Model file for the job. Use its own axes, mm. Face numbers are marked on the shaded views. A direction names the side the tool comes from. Round coordinates to 2 decimals unless told otherwise and drop trailing zeros. Order: outer loops, then holes, each group sorted by start corner. A loop starts at its lowest first (then second) coordinate and runs counter-clockwise, first axis right, second up. Notation, with made-up numbers: (-40, 44.25) - (7, 44.25) arc R12 cw to (7, 55.25) - close; hole circle Ø6 at (5, 13.25). An arc over 180 degrees is marked (long way). Write item = value, one per line. Start each with the question number.
from build123d import *

# Parameters (mm, degrees)
SKETCH_2_W          = 75
SKETCH_2_H          = 40
EXTRUDE_1_DEPTH     = 2
SKETCH_3_R          = 5.05
SKETCH_3_R_2        = 1.25
CUT_EXTRUDE_1_DEPTH = 86.023526156
FILLET_1_R          = 20
SKETCH_7_W          = 2
SKETCH_7_H          = 40
EXTRUDE_3_DEPTH     = 12
SKETCH_8_R          = 1.5
CUT_EXTRUDE_2_DEPTH = 10


with BuildPart() as part:
    # 草图2 → 凸台-拉伸1 (new body)
    with BuildSketch(Plane.XY):
        with Locations((37.5, 20)):
            Rectangle(SKETCH_2_W, SKETCH_2_H)
    extrude(amount=EXTRUDE_1_DEPTH)

    # 草图3 → 切除-拉伸1 (cut, through all)
    with BuildSketch(Plane(origin=(0, 0, 0), x_dir=(-1, 0, 0), z_dir=(0, 0, -1))):
        with Locations((-26, 20)):
            Circle(SKETCH_3_R)
        with Locations((-16, 10.202041029)):
            Circle(SKETCH_3_R_2)
    extrude(amount=-CUT_EXTRUDE_1_DEPTH, mode=Mode.SUBTRACT)

    # 圆角1
    fillet_1_edges = [part.edges().sort_by_distance(p)[0] for p in [
        (0, 40, 1),
        (0, 0, 1),
    ]]
    fillet(fillet_1_edges, radius=FILLET_1_R - 0.0001)  # a hair under: the kernel refuses the full size

    # 草图7 → 凸台-拉伸3 (add)
    with BuildSketch(Plane(origin=(0, 0, 0), x_dir=(-1, 0, 0), z_dir=(0, 0, -1))):
        with Locations((-74, 20)):
            Rectangle(SKETCH_7_W, SKETCH_7_H)
    extrude(amount=-EXTRUDE_3_DEPTH)

    # 草图8 → 切除-拉伸2 (cut)
    with BuildSketch(Plane.ZY.offset(-73)):
        with Locations((7, 33)):
            Circle(SKETCH_8_R)
        with Locations((7, 8)):
            Circle(SKETCH_8_R)
    extrude(amount=-CUT_EXTRUDE_2_DEPTH, mode=Mode.SUBTRACT)


solid = part.part
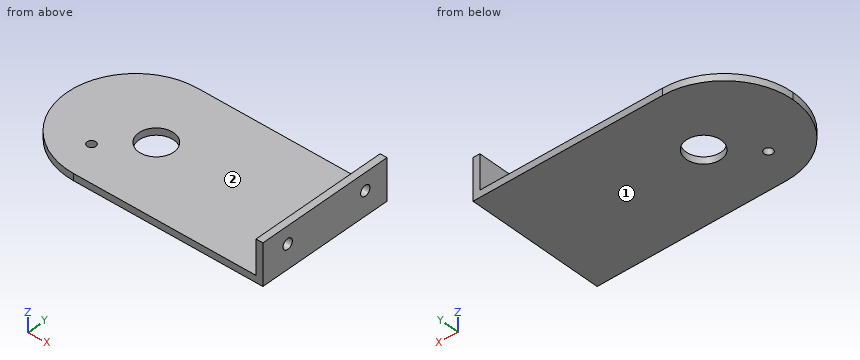
Item 1: Saw through at B-B, the plane z = 7. Give the cut face in (x, y), then the cut area to 3 significant figures.
Item 2: Saw through at A-A, the plane x = 26. Give the cut face in (y, z).
Item 3: Saw through at D-D, the plane z = 0.75. Give the number of separate pieces and of enclosed holes in the cut face, then the cut area to 3 significant figures.
Item 4: Probe L1, parallel to Y at x = 73.8, z = 7; L2, parallel to Z at x = 4, y = 24.5; L3, parallel to X at y = 10, z = 5. List the from-to ranges inside material, lowest first.
Item 5: Which spindle directions (+Z, -Z, +X, -X, +Y, -Y) get a long thin tool onto all of the face, cutting with end or side? Do the marked faces 1 and 2. Say none if no direction does.
Item 6: Drop flat-ended pins along their axis: pin 1 (1 mm diameter, centred on x = 17.5, z = 3, fed in from -Y); pin 2 (3 mm diameter, centred on x = 16, y = 10.2, fed in from +Z); pin 3 (4 mm diameter, centred on y = 8, z = 7, fed in from -X). Give the stop position or say it passes through.
Item 7: Saw through at C-C, the plane y = 33. Give the cut face in (x, z).
Check sheet entries:
q1.outline = (73, 0) - (75, 0) - (75, 6.5) - (73, 6.5) - close; (73, 9.5) - (75, 9.5) - (75, 31.5) - (73, 31.5) - close; (73, 34.5) - (75, 34.5) - (75, 40) - (73, 40) - close
q1.area = 68.0 mm2
q2.outline = (0, 0) - (14.95, 0) - (14.95, 2) - (0, 2) - close; (25.05, 0) - (40, 0) - (40, 2) - (25.05, 2) - close
q3.separate_pieces = 1
q3.enclosed_holes = 2
q3.area = 2,740 mm2
q4.L1 = 0 to 6.5, 9.5 to 31.5, 34.5 to 40
q4.L2 = 0 to 2
q4.L3 = 73 to 75
q5.face_1 = -Z, +X, -X, +Y, -Y
q5.face_2 = +Z, -X, +Y, -Y
q6.pin_1 = through
q6.pin_2 = 2
q6.pin_3 = 73
q7.outline = (4.8, 0) - (75, 0) - (75, 5.5) - (73, 5.5) - (73, 2) - (4.8, 2) - close; (73, 8.5) - (75, 8.5) - (75, 12) - (73, 12) - close
